Geometry check sheet. Reference: the model listing, model coordinates, mm. Face numbers are marked on the shaded views. A direction names the side the tool comes from. Give positions to 0.01 mm unless a question says otherwise; leave off trailing zeros. Loops run counter-clockwise (first coordinate to the right, second up) from the corner with the lowest first, then second, coordinate; pieces in that order, holes last. Notation, with made-up numbers: (57.25, -8) - (78.25, -8) arc R11 ccw to (78.25, 6) - close; hole circle Ø11 at (-5, 84.25). An arc over 180 degrees is marked (long way). Use a Markdown table: item, result. Add a question column.
1. Material ranges on L1, parallel to X at y = 3.75, z = 0 (3 decimals); L2, parallel to Z at x = 0.5, y = 4.25; L3, parallel to Z at x = -1, y = 5, recorded low to high.
2. Cross-section at C-C on y = 6.5. Enter the section's corners in (x, z) (3 decimals), and give its area (3 significant figures).
3. Cross-section at B-B on x = 12. Enter the section's corners in (y, z), and give its area (3 significant figures).
4. Depth check by flat-ended pin: P1, Ø1, axis at x = 3, y = 3, coming from the +Z side; P2, Ø2.5, axis at x = 12, z = 0, coming from the +Y side; P3, Ø1, axis at y = 3, z = -7.5, coming from the -X side; P4, Ø1, axis at y = 6.5, z = 10.5, coming from the -X side. Enter the tip coordinate at first touch or a pass-through.
5. Set-up check for the marked faces 4 and 5: record each of +Z, -Z, +X, -X, +Y, -Y from which the full face is reachable in a straight line by a thin tool's end or side.
6. Draft check along Z on the marked faces 1, 2 and 3. Enter one of: pulls with the +Z half, pulls with the -Z half, needs draft (parallel to the pull), parting line crosses it, or undercut.
7. Cross-section at A-A on z = -12. Enter the section's corners in (x, y).
from build123d import *

# Parameters (mm, degrees)
SKETCH1_R               = 15
SKETCH1_R_2             = 4.125
SKETCH1_R_3             = 1.5
BOSS_EXTRUDE1_DEPTH     = 8.6
CUT_EXTRUDE1_DEPTH      = 8.6
CUT_EXTRUDE2_DEPTH      = 8.6
CUT_EXTRUDE2_DEPTH_BACK = 30
SKETCH3_R               = 1.5


with BuildPart() as part:
    # Sketch1 → Boss-Extrude1 (new body)
    with BuildSketch(Plane(origin=(0, 0, 0), x_dir=(1, 0, 0), z_dir=(0, 1, 0))):
        with Locations(Location((0, 0, 0), (0, 0, 90))):
            Circle(SKETCH1_R)
        with Locations(Location((0, 0, 0), (0, 0, 90))):
            Circle(SKETCH1_R_2, mode=Mode.SUBTRACT)
        with Locations(Location((0, 12, 0), (0, 0, 90))):
            Circle(SKETCH1_R_3, mode=Mode.SUBTRACT)
        with Locations(Location((12, 0, 0), (0, 0, 90))):
            Circle(SKETCH1_R_3, mode=Mode.SUBTRACT)
        with Locations(Location((0, -12, 0), (0, 0, 90))):
            Circle(SKETCH1_R_3, mode=Mode.SUBTRACT)
        with Locations(Location((-12, 0, 0), (0, 0, 90))):
            Circle(SKETCH1_R_3, mode=Mode.SUBTRACT)
    extrude(amount=BOSS_EXTRUDE1_DEPTH)

    # Sketch2 → Cut-Extrude1 (cut)
    with BuildSketch(Plane(origin=(0, 8.6, 0), x_dir=(1, 0, 0), z_dir=(0, 1, 0))):
        Polygon((8.202438662, 8.202438662), (6.187184335, 10.217692988), (4.348706704, 8.379215357), (8.379215357, 4.348706704), (10.217692988, 6.187184335), align=None)
        Polygon((-10.217692988, -6.187184335), (-8.379215357, -4.348706704), (-4.348706704, -8.379215357), (-6.187184335, -10.217692988), (-8.202438662, -8.202438662), align=None)
    extrude(amount=-CUT_EXTRUDE1_DEPTH, mode=Mode.SUBTRACT)

    # Sketch3 → Cut-Extrude2 (cut, two sides: drawn at the far end of the back side and taken through both)
    with BuildSketch(Plane(origin=(6.363961031, 0, -6.363961031), x_dir=(-0.7071067811865489, 0, -0.7071067811865461), z_dir=(0.7071067811865461, 0, -0.7071067811865489)).offset(-CUT_EXTRUDE2_DEPTH_BACK)):
        with Locations(Location((0, 4.3, 0), (0, 0, 180))):
            Circle(SKETCH3_R)
    extrude(amount=CUT_EXTRUDE2_DEPTH + CUT_EXTRUDE2_DEPTH_BACK, mode=Mode.SUBTRACT)


solid = part.part
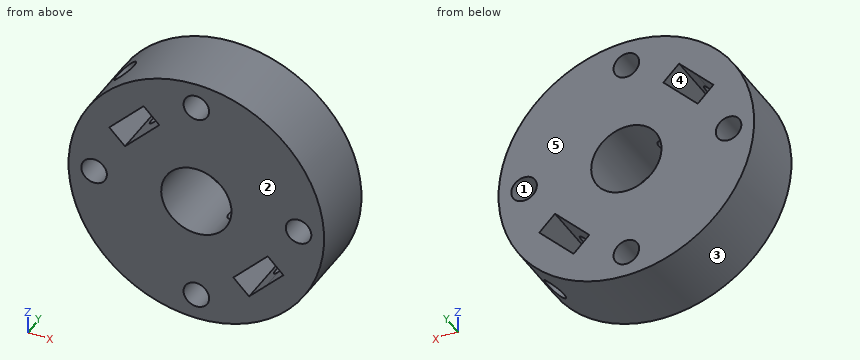
Values found:
| question | item | result |
|---|---|---|
| 1 | L1 | x = -15 to -13.5, -10.5 to -4.125, 4.125 to 10.5, 13.5 to 15 |
| 1 | L2 | z = -14.99 to -13.41, -10.59 to -4.09, 4.09 to 10.59, 13.41 to 14.99 |
| 1 | L3 | z = -14.97 to -13.12, -10.88 to -4, 4 to 10.88, 13.12 to 14.97 |
| 2 | outline | circle Ø30 at (0, 0); hole circle Ø3 at (-12, 0); hole (-10.218, 6.187) - (-8.379, 4.349) - (-4.349, 8.379) - (-6.187, 10.218) - close; hole circle Ø8.25 at (0, 0); hole circle Ø3 at (0, -12); hole circle Ø3 at (0, 12); hole (4.349, -8.379) - (6.187, -10.218) - (10.218, -6.187) - (8.379, -4.349) - close; hole circle Ø3 at (12, 0) |
| 2 | area | 595 mm2 |
| 3 | outline | (0, -9) - (8.6, -9) - (8.6, -1.5) - (0, -1.5) - close; (0, 1.5) - (8.6, 1.5) - (8.6, 9) - (0, 9) - close |
| 3 | area | 129 mm2 |
| 4 | P1 | stops at z = 14.79 |
| 4 | P2 | passes through |
| 4 | P3 | stops at x = -13.27 |
| 4 | P4 | stops at x = -11.18 |
| 5 | face 4 | +Y, -Y |
| 5 | face 5 | +Z, -Z, +X, -X, +Y |
| 6 | face 1 | undercut |
| 6 | face 2 | needs draft |
| 6 | face 3 | parting line crosses it |
| 7 | outline | (-9, 0) - (-1.5, 0) - (-1.5, 8.6) - (-9, 8.6) - close; (1.5, 0) - (9, 0) - (9, 8.6) - (1.5, 8.6) - close |
